Autodesk Inventor part; units mm, degrees
ref_plane "YZ Plane" through (0, 0, 0) normal (1, 0, 0) x (0, 1, 0)
ref_plane "XZ Plane" through (0, 0, 0) normal (0, 1, 0) x (-1, 0, 0)
ref_plane "XY Plane" through (0, 0, 0) normal (0, 0, 1) x (1, 0, 0)
sketch "Schizzo1" plane through (0, 0, 0) normal (0, 1, 0) x (-1, 0, 0)
  line L0 (5, 5) -> (-5, 5)
  line L1 (-5, 5) -> (-5, -5)
  line L2 (-5, -5) -> (5, -5)
  line L3 (5, -5) -> (5, 5)
  line L4 (10, 10) -> (-10, 10)
  line L5 (-10, 10) -> (-10, -10)
  line L6 (-10, -10) -> (10, -10)
  line L7 (10, -10) -> (10, 10)
  line L8 (0, 0) -> (14, 0) construction
  line L9 (0, 0) -> (0, -16.4941) construction
  line L10 (10, 10) -> (18, 10)
  line L11 (18, 10) -> (18, 5)
  line L12 (18, 5) -> (10, 5)
  line L13 (10, -10) -> (18, -10)
  line L14 (18, -10) -> (18, -5)
  line L15 (18, -5) -> (10, -5)
  line L16 (-10, 10) -> (-18, 10)
  line L17 (-18, 10) -> (-18, 5)
  line L18 (-18, 5) -> (-10, 5)
  line L19 (-10, -10) -> (-18, -10)
  line L20 (-18, -10) -> (-18, -5)
  line L21 (-18, -5) -> (-10, -5)
  dimension "d0" = 20
  dimension "d1" = 10
  dimension "d2" = 8
  dimension "d3" = 5
extrude "Estrusione1" add sketch "Schizzo1" along normal blind 10 and the other way blind 35 contours L7 L6 L5 L4
extrude "Estrusione2" add sketch "Schizzo1" along normal blind 10 contours L10 L11 L12 L7 | L5 L18 L17 L16 | L15 L14 L13 L7 | L5 L19 L20 L21
fillet "Raccordo1" radius 8 4 edges at (10, 0, 7.5) (10, 0, -7.5) (-10, 0, -7.5) (-10, 0, 7.5)
sketch "Schizzo2" plane through (0, 0, 0) normal (0, 0, 1) x (1, 0, 0)
  line L0 (-18, 0) -> (-18, 10)
  line L1 (-18, 10) -> (18, 10)
  line L2 (18, 0) -> (18, 10)
  arc A0 (18, 0) -> (10, -8) centre (18, -8) ccw
  arc A1 (-10, -8) -> (-18, 0) centre (-18, -8) ccw
  line L3 (-10, -8) -> (-10, 10)
  line L4 (10, 10) -> (10, -8)
  circle A2 centre (-14, 5) radius 2.75
  line L5 (0, 0) -> (0, 11.3165) construction
  circle A3 centre (14, 5) radius 2.75
  dimension "d11" = 5.5
  dimension "d12" = 5
  dimension "d13" = 4
extrude "Estrusione3" cut sketch "Schizzo2" along normal through all both and the other way through all contours A2 | A3
equation "\"RaggioPiega\" = Spessore"
equation "\"LarghezzaScaricoPiega\" = Spessore"
equation "\"ProfonditàScaricoPiega\" = 0.5 * Spessore"
equation "\"DimensioniScaricoAngolo\" = 4 * Spessore"
equation "\"ResiduoMinimo\" = 2 * Spessore"
equation "\"RaggioTransizione\" = RaggioPiega"
equation "\"Dimensione_raggio_Jacobi\" = RaggioPiega"
equation "\"DimensioneGioco\" = Spessore"
properties part number "asta con serraggio pinza"
Geometry check sheet. Reference: the model listing, model coordinates, mm. A direction names the side the tool comes from. Coordinates: 2 decimals unless noted, no trailing zeros. Write each loop counter-clockwise with the first axis right and the second up, starting at its lowest first coordinate (ties: lowest second). Pieces come first, ordered by that corner, then holes. Notation, with made-up numbers: (59, 65.25) -> (80, 65.25) arc R10 ccw to (80, 76.25) -> close; hole circle Ø3 at (89.5, -14). An arc over 180 degrees is marked (long way). One line per question, with ' | ' between items.
1. Cross-section at C-C on y = 5. State how many separate pieces and enclosed holes the cut face has, and give its area (3 significant figures).
Answers:
separate pieces: 5 | enclosed holes: 1 | area: 350 mm²
2. Cross-section at B-B on x = 2.5. Record the cut outline in (y, z).
Answers:
outline: (-35, -10) -> (10, -10) -> (10, -5) -> (-35, -5) -> close; (-35, 5) -> (10, 5) -> (10, 10) -> (-35, 10) -> close
3. Cross-section at D-D on y = -9. Record the cut outline in (x, z).
Answers:
outline: (-10, -10) -> (10, -10) -> (10, 10) -> (-10, 10) -> close; hole (-5, -5) -> (5, -5) -> (5, 5) -> (-5, 5) -> close
4. Cross-section at A-A on z = -0.25. Record the cut outline in (x, y).
Answers:
outline: (-10, -35) -> (-5, -35) -> (-5, 10) -> (-10, 10) -> close; (5, -35) -> (10, -35) -> (10, 10) -> (5, 10) -> close
5. Thickness scan on probe 1 along X at (y, z) = (5, 7.35); probe 2 along X at (y, z) = (-32, -3.5). Record the ranges inside material, lowest first. Write a range as from..to.
Answers:
probe 1: x = -18..-16.75, -11.25..11.25, 16.75..18 | probe 2: x = -10..-5, 5..10
6. Set-up check for faces 1 (the flat face through (-10, -18, 0)), 2 (the flat face through (5, -13, 0)), 3 (the flat face through (-11, 3, 5)): record each of +Z, -Z, +X, -X, +Y, -Y from which the full face is reachable in a straight line by a thin tool's end or side.
Answers:
face 1: -X, -Y | face 2: +Y, -Y | face 3: -X, +Y, -Y
7. Depth check by flat-ended pin: pin 1 Ø4.5 at (x, y) = (-14, 5) entering from -Z; pin 2 Ø1.5 at (y, z) = (-14, 1.5) entering from +X; pin 3 Ø1 at (y, z) = (-23, 7.5) entering from -X. Enter the tip coordinate at first touch or a pass-through.
Answers:
pin 1: passes through | pin 2: stops at x = 10 | pin 3: stops at x = -10
8. Draft check along X on faces 4 (the flat face through (18, 5, 8)), 5 (the flat face through (0, -13, -5)), 6 (the flat face through (-18, 5, -8)). Enter one of: +X half, -X half, draft (parallel to the pull), parting line (faces both ways), or undercut.
Answers:
face 4: +X half | face 5: undercut | face 6: -X half
